Geometry: final body of the model. Coordinates: model frame, mm. Face numbers are marked on the shaded views. Coordinates: 2 decimals unless noted, no trailing zeros. Write each loop counter-clockwise with the first axis right and the second up, starting at its lowest first coordinate (ties: lowest second). Pieces come first, ordered by that corner, then holes. Notation, with made-up numbers: (45, 71) -> (92, 71) arc R20 ccw to (92, 97) -> close; hole circle Ø9 at (86.25, 19). An arc over 180 degrees is marked (long way). One line per item, written item: value. Start each with the question number.
from build123d import *

# Parameters (mm, degrees)
SKETCH1_W                = 2400
SKETCH1_H                = 225
BOSS_EXTRUDE1_DEPTH      = 10
BOSS_EXTRUDE4_START      = 30
BOSS_EXTRUDE4_DEPTH      = 80
BOSS_EXTRUDE5_START      = -30
BOSS_EXTRUDE5_DEPTH      = 80
BOSS_EXTRUDE6_DEPTH      = 105
BOSS_EXTRUDE6_DEPTH_BACK = 105


with BuildPart() as part:
    # Sketch1 → Boss-Extrude1 (new body)
    with BuildSketch(Plane(origin=(0, 0, 0), x_dir=(1, 0, 0), z_dir=(0, 1, 0))):
        Rectangle(SKETCH1_W, SKETCH1_H)
    extrude(amount=BOSS_EXTRUDE1_DEPTH)

    # Sketch8 → Boss-Extrude4 (add)
    with BuildSketch(Plane.XY.offset(BOSS_EXTRUDE4_START)):
        Polygon((425, 10), (450, 40), (575, 40), (600, 10), align=None)
    extrude(amount=BOSS_EXTRUDE4_DEPTH)

    # Sketch14 → Boss-Extrude5 (add)
    with BuildSketch(Plane.XY.offset(BOSS_EXTRUDE5_START)):
        Polygon((-75, 10), (100, 10), (75, 40), (-50, 40), align=None)
    extrude(amount=-BOSS_EXTRUDE5_DEPTH)

    # Sketch15 → Boss-Extrude6 (add, two sides)
    with BuildSketch(Plane.XY) as boss_extrude6_sk:
        Polygon((-400, 10), (-425, 40), (-550, 40), (-575, 10), align=None)
    extrude(amount=BOSS_EXTRUDE6_DEPTH)
    extrude(boss_extrude6_sk.sketch, amount=-BOSS_EXTRUDE6_DEPTH_BACK)


solid = part.part
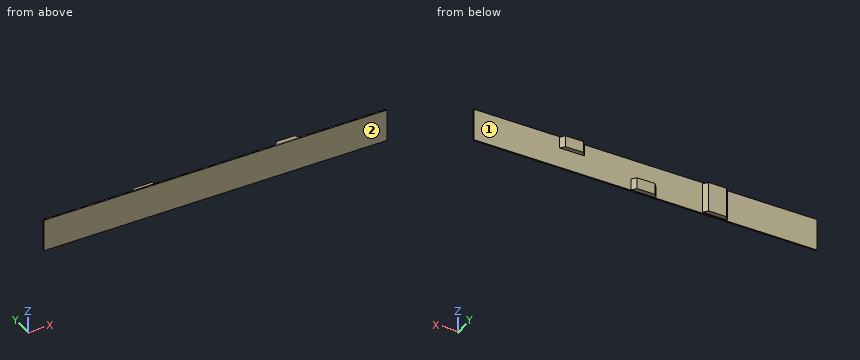
Q1. Cut plane D-D on x = -838.5. Output: boundary loops of the cut face in (y, z), and give its area (3 significant figures).
Q2. First-contact query: P1, Ø12, axis at x = -44.5, y = 18, coming from the -Z side; P2, Ø15, axis at x = 504.5, y = 19, coming from the -Z side; P3, Ø10, axis at x = 524, z = -60, coming from the +Y side. Flat tips, straight axial feed; report the tip coordinate or a pass-through.
Q3. Line query: L1, parallel to Y at x = -43.5, z = 23; L2, parallel to X at y = 30, z = -96; L3, parallel to X at y = 15, z = -47. Output: solid intervals per line, ascending. Write a range as from..to.
Q4. Cut plane C-C on x = -27. Output: boundary loops of the cut face in (y, z).
Q5. Draft query along X for the marked faces 1 and 2. Return one class per face: pulls with the +X half, pulls with the -X half, needs draft (parallel to the pull), parting line crosses it, or undercut.
Q6. Cut plane A-A on y = 23.5. Output: boundary loops of the cut face in (x, z), and give its area (3 significant figures).
Q7. Cut plane B-B on z = -71.5. Output: boundary loops of the cut face in (x, y).
Solution:
1. outline: (0, -112.5) -> (10, -112.5) -> (10, 112.5) -> (0, 112.5) -> close
1. area: 2,250 mm²
2. P1: z = -110
2. P2: z = 30
2. P3: y = 10
3. L1: 0..10
3. L2: -558.33..-416.67, -58.33..83.33
3. L3: -570.83..-404.17, -70.83..95.83
4. outline: (0, -112.5) -> (10, -112.5) -> (10, -110) -> (40, -110) -> (40, -30) -> (10, -30) -> (10, 112.5) -> (0, 112.5) -> close
5. face 1: undercut
5. face 2: needs draft
6. outline: (-563.75, -105) -> (-411.25, -105) -> (-411.25, 105) -> (-563.75, 105) -> close; (-63.75, -110) -> (88.75, -110) -> (88.75, -30) -> (-63.75, -30) -> close; (436.25, 30) -> (588.75, 30) -> (588.75, 110) -> (436.25, 110) -> close
6. area: 56,400 mm²
7. outline: (-1200, 0) -> (1200, 0) -> (1200, 10) -> (100, 10) -> (75, 40) -> (-50, 40) -> (-75, 10) -> (-400, 10) -> (-425, 40) -> (-550, 40) -> (-575, 10) -> (-1200, 10) -> close
